For this review, take the finished solid that the model builds, in its own axes (mm). Give positions to 0.01 mm unless a question says otherwise; leave off trailing zeros. Order: outer loops, then holes, each group sorted by start corner. A loop starts at its lowest first (then second) coordinate and runs counter-clockwise, first axis right, second up. Notation, with made-up numbers: (-24, 47.5) -> (18, 47.5) arc R30 ccw to (18, 81.5) -> close; hole circle Ø5 at (68, 60.5). An arc over 180 degrees is marked (long way). Return JSON: item names as keys, results as strings. Group by question number.
1) The part is to be moulded in two halves that separate along Y. For faces 1 (the face through (123.16, 29.66, 0.91)), 2 (the face through (123.06, -29.76, 0.91)), 3 (the face through (-121.45, 16.265, 0.94)), say which applies: released by +Y, released by -Y, zero draft, split by the parting line, or undercut.
2) To check wall thickness, follow line 1 along Y through (x, z) = (15.5, 1.1); line 2 along Y through (x, z) = (-79, 0.8); line 3 along X through (y, z) = (16.5, 1.35). State the ranges of each line that lie inside material, in increasing order.
3) Add section B-B (x = 75). Give the boundary of the cut face in (y, z), then the cut area to 3 significant figures.
4) Insertion check: P1, Ø0.9, axis at y = 4.5, z = 1.5, coming from the +X side. The pin has a flat end and moves straight along its axis. Give the tip position at first contact, or say it passes through.
5) Add section A-A (x = -86). Give the boundary of the cut face in (y, z), then the cut area to 3 significant figures.
6) Add section C-C (y = -3). State how many separate pieces and enclosed holes the cut face has, then the cut area to 3 significant figures.
from build123d import *

# Parameters (mm, degrees)
MAINBODY_DEPTH    = 1.8542
SKETCH3_R         = 1.9685
MOUNTHOLES_DEPTH  = 2.8542
PANELCUTOUT_REACH = 3.854
SKETCH4_W         = 40.934
SKETCH4_H         = 7.854
SKETCH4_W_2       = 57.654
SKETCH4_H_2       = 7.254
SKETCH4_W_3       = 8.654


with BuildPart() as part:
    # Sketch2 → MainBody (new body)
    with BuildSketch(Plane.XY):
        with BuildLine():
            Line((118.618, 31.5722), (-118.618, 31.5722))
            ThreePointArc((-118.618, 31.5722), (-123.108128061, 29.712328061), (-124.968, 25.2222))
            Line((-124.968, 25.2222), (-124.968, 9.9822))
            Line((-124.968, 9.9822), (-121.793, 9.9822))
            Line((-121.793, 9.9822), (-121.793, -9.9822))
            Line((-121.793, -9.9822), (-124.968, -9.9822))
            Line((-124.968, -9.9822), (-124.968, -25.2222))
            ThreePointArc((-124.968, -25.2222), (-123.108128061, -29.712328061), (-118.618, -31.5722))
            Line((-118.618, -31.5722), (118.618, -31.5722))
            ThreePointArc((118.618, -31.5722), (123.108128061, -29.712328061), (124.968, -25.2222))
            Line((124.968, -25.2222), (124.968, -9.9822))
            Line((124.968, -9.9822), (121.793, -9.9822))
            Line((121.793, -9.9822), (121.793, 9.9822))
            Line((121.793, 9.9822), (124.968, 9.9822))
            Line((124.968, 9.9822), (124.968, 25.2222))
            ThreePointArc((124.968, 25.2222), (123.108128061, 29.712328061), (118.618, 31.5722))
        make_face()
    extrude(amount=MAINBODY_DEPTH)

    # Sketch3 → MountHoles (cut, through all)
    with BuildSketch(Plane.XY.offset(1.8542)):
        with Locations((-119.888, 17.4625)):
            Circle(SKETCH3_R)
        with Locations((119.888, 17.4625)):
            Circle(SKETCH3_R)
        with Locations((119.888, -17.4625)):
            Circle(SKETCH3_R)
        with Locations((-119.888, -17.4625)):
            Circle(SKETCH3_R)
    extrude(amount=-MOUNTHOLES_DEPTH, mode=Mode.SUBTRACT)

    # Sketch4 → PanelCutout (cut, up to next)
    with BuildSketch(Plane.XY.offset(1.8542), mode=Mode.PRIVATE) as panelcutout_sk1:
        with BuildLine():
            Line((51.153291776, -12.65754977), (57.304708224, -12.65754977))
            ThreePointArc((57.304708224, -12.65754977), (54.229, -0.64334977), (51.153291776, -12.65754977))
        make_face()
    panelcutout_tool1 = extrude(panelcutout_sk1.sketch, amount=-PANELCUTOUT_REACH, mode=Mode.PRIVATE) & part.part
    add(panelcutout_tool1.solids().sort_by_distance((54.229, -6.889516, 1.8542))[0], mode=Mode.SUBTRACT)
    # Sketch4 → PanelCutout (cut, up to next)
    with BuildSketch(Plane.XY.offset(1.8542), mode=Mode.PRIVATE) as panelcutout_sk2:
        with Locations((89.535, -4.72055)):
            Rectangle(SKETCH4_W, SKETCH4_H)
    panelcutout_tool2 = extrude(panelcutout_sk2.sketch, amount=-PANELCUTOUT_REACH, mode=Mode.PRIVATE) & part.part
    add(panelcutout_tool2.solids().sort_by_distance((89.535, -4.72055, 1.8542))[0], mode=Mode.SUBTRACT)
    # Sketch4 → PanelCutout (cut, up to next)
    with BuildSketch(Plane.XY.offset(1.8542), mode=Mode.PRIVATE) as panelcutout_sk3:
        with BuildLine():
            Line((32.103291776, -12.65754977), (38.254708224, -12.65754977))
            ThreePointArc((38.254708224, -12.65754977), (35.179, -0.64334977), (32.103291776, -12.65754977))
        make_face()
    panelcutout_tool3 = extrude(panelcutout_sk3.sketch, amount=-PANELCUTOUT_REACH, mode=Mode.PRIVATE) & part.part
    add(panelcutout_tool3.solids().sort_by_distance((35.179, -6.889516, 1.8542))[0], mode=Mode.SUBTRACT)
    # Sketch4 → PanelCutout (cut, up to next)
    with BuildSketch(Plane.XY.offset(1.8542), mode=Mode.PRIVATE) as panelcutout_sk4:
        with BuildLine():
            Line((13.053291776, -12.65754977), (19.204708224, -12.65754977))
            ThreePointArc((19.204708224, -12.65754977), (16.129, -0.64334977), (13.053291776, -12.65754977))
        make_face()
    panelcutout_tool4 = extrude(panelcutout_sk4.sketch, amount=-PANELCUTOUT_REACH, mode=Mode.PRIVATE) & part.part
    add(panelcutout_tool4.solids().sort_by_distance((16.129, -6.889516, 1.8542))[0], mode=Mode.SUBTRACT)
    # Sketch4 → PanelCutout (cut, up to next)
    with BuildSketch(Plane.XY.offset(1.8542), mode=Mode.PRIVATE) as panelcutout_sk5:
        with BuildLine():
            Line((-5.996708224, -12.65754977), (0.154708224, -12.65754977))
            ThreePointArc((0.154708224, -12.65754977), (-2.921, -0.64334977), (-5.996708224, -12.65754977))
        make_face()
    panelcutout_tool5 = extrude(panelcutout_sk5.sketch, amount=-PANELCUTOUT_REACH, mode=Mode.PRIVATE) & part.part
    add(panelcutout_tool5.solids().sort_by_distance((-2.921, -6.889516, 1.8542))[0], mode=Mode.SUBTRACT)
    # Sketch4 → PanelCutout (cut, up to next)
    with BuildSketch(Plane.XY.offset(1.8542), mode=Mode.PRIVATE) as panelcutout_sk6:
        with BuildLine():
            Line((-25.046708224, -12.65754977), (-18.895291776, -12.65754977))
            ThreePointArc((-18.895291776, -12.65754977), (-21.971, -0.64334977), (-25.046708224, -12.65754977))
        make_face()
    panelcutout_tool6 = extrude(panelcutout_sk6.sketch, amount=-PANELCUTOUT_REACH, mode=Mode.PRIVATE) & part.part
    add(panelcutout_tool6.solids().sort_by_distance((-21.971, -6.889516, 1.8542))[0], mode=Mode.SUBTRACT)
    # Sketch4 → PanelCutout (cut, up to next)
    with BuildSketch(Plane.XY.offset(1.8542), mode=Mode.PRIVATE) as panelcutout_sk7:
        with Locations((-68.171, -4.42055)):
            Rectangle(SKETCH4_W_2, SKETCH4_H_2)
    panelcutout_tool7 = extrude(panelcutout_sk7.sketch, amount=-PANELCUTOUT_REACH, mode=Mode.PRIVATE) & part.part
    add(panelcutout_tool7.solids().sort_by_distance((-68.171, -4.42055, 1.8542))[0], mode=Mode.SUBTRACT)
    # Sketch4 → PanelCutout (cut, up to next)
    with BuildSketch(Plane.XY.offset(1.8542), mode=Mode.PRIVATE) as panelcutout_sk8:
        with Locations((-105.5650001, -4.42055)):
            Rectangle(SKETCH4_W_3, SKETCH4_H_2)
    panelcutout_tool8 = extrude(panelcutout_sk8.sketch, amount=-PANELCUTOUT_REACH, mode=Mode.PRIVATE) & part.part
    add(panelcutout_tool8.solids().sort_by_distance((-105.565, -4.42055, 1.8542))[0], mode=Mode.SUBTRACT)


solid = part.part
Evaluation:
{
 "1": {"face 1": "released by +Y", "face 2": "released by -Y", "face 3": "undercut"},
 "2": {"line 1": "-31.57 to -12.66, -0.67 to 31.57", "line 2": "-31.57 to -8.05, -0.79 to 31.57", "line 3": "-124.97 to -121.61, -118.17 to 118.17, 121.61 to 124.97"},
 "3": {"outline": "(-31.57, 0) -> (-8.65, 0) -> (-8.65, 1.85) -> (-31.57, 1.85) -> close; (-0.79, 0) -> (31.57, 0) -> (31.57, 1.85) -> (-0.79, 1.85) -> close", "area": "103 mm^2"},
 "4": {"P1": "x = 121.79"},
 "5": {"outline": "(-31.57, 0) -> (-8.05, 0) -> (-8.05, 1.85) -> (-31.57, 1.85) -> close; (-0.79, 0) -> (31.57, 0) -> (31.57, 1.85) -> (-0.79, 1.85) -> close", "area": "104 mm^2"},
 "6": {"separate pieces": "9", "enclosed holes": "0", "area": "161 mm^2"}
}
